The model under review builds one solid part; all positions refer to its coordinate system, in mm. Face numbers are marked on the shaded views. A direction names the side the tool comes from. Round coordinates to 2 decimals unless told otherwise and drop trailing zeros. Write each loop counter-clockwise with the first axis right and the second up, starting at its lowest first coordinate (ties: lowest second). Pieces come first, ordered by that corner, then holes. Notation, with made-up numbers: M 27.25,-19 L 39.25,-19 A13 cw 39.25,-6 Z; hole C 48,24.25 d7. An arc over 180 degrees is marked long. One line per item, written item: value. Start each with the question number.
1) Mouldability with a two-part tool opening along Y and no side actions: class the marked faces 1, 2 and 3 as +Y half, -Y half, draft (parallel to the pull), parting line (faces both ways), or undercut.
2) Take a section at A-A, the plane x = 0. Write out the cut boundary in (y, z).
3) Take a section at B-B, the plane z = -8.25. Write out the cut boundary in (x, y), and give its area (3 significant figures).
4) Wall thickness on probe 1 along Y at (x, z) = (0, 5.5); probe 2 along Y at (x, z) = (-6.5, -8.5); probe 3 along Y at (x, z) = (10, -10.5): over which ranges is each line inside the solid? List them lowest first.
5) For P1, Ø3, axis at x = 21.5, y = 4, coming from the +Z side; P2, Ø6, axis at x = 20, y = -9.5, coming from the -Z side; P3, Ø8, axis at y = -27, z = 5.5, coming from the -X side; P4, Ø8, axis at x = 0, y = 0, coming from the +Z side, all flat-tipped, find the tip position at first contact; note any pin that passes through.
6) Tool access review of the marked faces 4, 5 and 6: name each direction out of +Z, -Z, +X, -X, +Y, -Y from which nothing blocks a thin tool from reaching the whole face with its end or side.
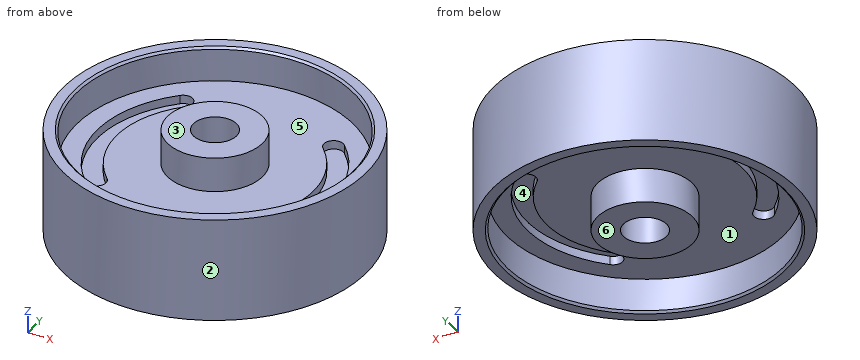
from build123d import *

# Parameters (mm, degrees)
SKETCH_1_R               = 35
EXTRUDE_1_DEPTH          = 12
CUT_EXTRUDE_1_DEPTH      = 51.931326313
CUT_EXTRUDE_1_DEPTH_BACK = 51.931326313
SKETCH_2_R               = 5
SKETCH_3_R               = 32
SKETCH_3_R_2             = 11
CUT_EXTRUDE_2_DEPTH      = 8
CUT_EXTRUDE_3_DEPTH      = 2
CHAMFER_1_SIZE           = 0.5


with BuildPart() as part:
    # 草图1 → 凸台-拉伸1 (new, symmetric)
    with BuildSketch(Plane.XY):
        Circle(SKETCH_1_R)
    extrude(amount=EXTRUDE_1_DEPTH, both=True)

    # 草图2 → 切除-拉伸1 (cut, two sides: drawn at the far end of the back side and taken through both)
    with BuildSketch(Plane.XY.offset(-CUT_EXTRUDE_1_DEPTH_BACK)):
        Circle(SKETCH_2_R)
    extrude(amount=CUT_EXTRUDE_1_DEPTH + CUT_EXTRUDE_1_DEPTH_BACK, mode=Mode.SUBTRACT)

    # 草图3 → 切除-拉伸2 (cut)
    with BuildSketch(Plane.XY.offset(12)):
        Circle(SKETCH_3_R)
        Circle(SKETCH_3_R_2, mode=Mode.SUBTRACT)
    cut_extrude_2 = extrude(amount=-CUT_EXTRUDE_2_DEPTH, mode=Mode.SUBTRACT)

    # 草图4 → 切除-拉伸3 (cut)
    with BuildSketch(Plane.XY.offset(4)):
        with BuildLine():
            ThreePointArc((-19.268659787, 19.268659787), (-27.25, 0), (-19.268659787, -19.268659787))
            ThreePointArc((-19.268659787, -19.268659787), (-16.086679272, -19.268659787), (-16.086679272, -16.086679272))
            ThreePointArc((-16.086679272, -16.086679272), (-22.75, 0), (-16.086679272, 16.086679272))
            ThreePointArc((-16.086679272, 16.086679272), (-16.086679272, 19.268659787), (-19.268659787, 19.268659787))
        make_face()
        with BuildLine():
            ThreePointArc((19.268659787, 19.268659787), (27.25, 0), (19.268659787, -19.268659787))
            ThreePointArc((19.268659787, -19.268659787), (16.086679272, -19.268659787), (16.086679272, -16.086679272))
            ThreePointArc((16.086679272, -16.086679272), (22.75, 0), (16.086679272, 16.086679272))
            ThreePointArc((16.086679272, 16.086679272), (16.086679272, 19.268659787), (19.268659787, 19.268659787))
        make_face()
    cut_extrude_3 = extrude(amount=-CUT_EXTRUDE_3_DEPTH, mode=Mode.SUBTRACT)

    # 镜向1: 切除-拉伸2, 切除-拉伸3 across plane
    add(cut_extrude_2.mirror(Plane.XY), mode=Mode.SUBTRACT)
    add(cut_extrude_3.mirror(Plane.XY), mode=Mode.SUBTRACT)

    # 倒角1
    chamfer_1_edges = [part.edges().sort_by_distance(p)[0] for p in [
        (-32, 0, 12),
        (-32, 0, -12),
    ]]
    chamfer(chamfer_1_edges, length=CHAMFER_1_SIZE)


solid = part.part
Checked values:
1. face 1: undercut
1. face 2: parting line
1. face 3: draft
2. outline: M -35,-12 L -32.5,-12 L -32,-11.5 L -32,-4 L -11,-4 L -11,-12 L -5,-12 L -5,12 L -11,12 L -11,4 L -32,4 L -32,11.5 L -32.5,12 L -35,12 Z; M 5,-12 L 11,-12 L 11,-4 L 32,-4 L 32,-11.5 L 32.5,-12 L 35,-12 L 35,12 L 32.5,12 L 32,11.5 L 32,4 L 11,4 L 11,12 L 5,12 Z
3. outline: C 0,0 d70; C 0,0 d22; hole C 0,0 d64; hole C 0,0 d10
3. area: 933 mm2
4. probe 1: y = -35 to -32, -11 to -5, 5 to 11, 32 to 35
4. probe 2: y = -34.39 to -31.33, -8.87 to 8.87, 31.33 to 34.39
4. probe 3: y = -33.54 to -30.4, -4.58 to 4.58, 30.4 to 33.54
5. P1: stops at z = 4
5. P2: stops at z = -4
5. P3: stops at x = -26.38
5. P4: passes through
6. face 4: -Z
6. face 5: +Z
6. face 6: -Z, +X, -X, +Y, -Y
